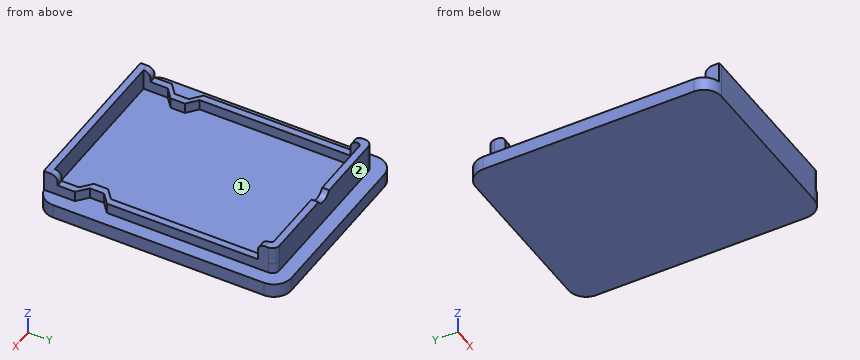
from build123d import *

# Parameters (mm, degrees)
PAD_DEPTH    = 2
PAD001_DEPTH = 1.5
PAD002_DEPTH = 1.5
PAD003_DEPTH = 2.5
SKETCH004_R  = 1.5
POCKET_DEPTH = 5
FILLET_R     = 1
FILLET001_R  = 1
FILLET002_R  = 1


with BuildPart() as part:
    # Sketch → Pad (new body)
    with BuildSketch(Plane.XY):
        with BuildLine():
            Line((-11.5, 17.5), (11.5, 17.5))
            ThreePointArc((14, 15), (13.267767, 16.767767), (11.5, 17.5))
            Line((14, 15), (14, -15))
            ThreePointArc((11.5, -17.5), (13.267767, -16.767767), (14, -15))
            Line((11.5, -17.5), (-11.5, -17.5))
            ThreePointArc((-14, -15), (-13.267767, -16.767767), (-11.5, -17.5))
            Line((-14, -15), (-14, 15))
            ThreePointArc((-11.5, 17.5), (-13.267767, 16.767767), (-14, 15))
        make_face()
    extrude(amount=PAD_DEPTH)

    # Sketch001 (on Face10 of Pad) → Pad001 (join)
    with BuildSketch(Plane.XY.offset(2)):
        with BuildLine():
            Line((-11, 15.5), (11, 15.5))
            ThreePointArc((12, 14.5), (11.707107, 15.207107), (11, 15.5))
            Line((12, 14.5), (12, -8.5))
            Line((12, -8.5), (10.5, -9.76))
            Line((10.5, -9.76), (10.5, -11.79))
            Line((10.5, -11.79), (12, -13.05))
            Line((12, -13.05), (12, -17.44949))
            ThreePointArc((11.5, -17.5), (11.751272, -17.48734), (12, -17.44949))
            Line((-11.5, -17.5), (11.5, -17.5))
            ThreePointArc((-12, -17.44949), (-11.751272, -17.48734), (-11.5, -17.5))
            Line((-12, -13.05), (-12, -17.44949))
            Line((-10.5, -11.79), (-12, -13.05))
            Line((-10.5, -9.76), (-10.5, -11.79))
            Line((-12, -8.5), (-10.5, -9.76))
            Line((-12, 14.5), (-12, -8.5))
            ThreePointArc((-11, 15.5), (-11.707107, 15.207107), (-12, 14.5))
        make_face()
        with BuildLine():
            Line((-11, -16.5), (-11, -13.05))
            Line((-11, -13.05), (-9.5, -11.79))
            Line((-9.5, -11.79), (-9.5, -9.76))
            Line((-9.5, -9.76), (-11, -8.5))
            Line((-11, -8.5), (-11, 14))
            ThreePointArc((-10.5, 14.5), (-10.853553, 14.353553), (-11, 14))
            Line((-10.5, 14.5), (10.5, 14.5))
            ThreePointArc((11, 14), (10.853553, 14.353553), (10.5, 14.5))
            Line((11, 14), (11, -8.5))
            Line((11, -8.5), (9.5, -9.76))
            Line((9.5, -9.76), (9.5, -11.79))
            Line((9.5, -11.79), (11, -13.05))
            Line((11, -13.05), (11, -16.5))
            Line((11, -16.5), (-11, -16.5))
        make_face(mode=Mode.SUBTRACT)
    extrude(amount=PAD001_DEPTH)

    # Sketch002 (on Face26 of Pad001) → Pad002 (join)
    with BuildSketch(Plane.XY.offset(3.5)):
        with BuildLine():
            ThreePointArc((11.5, -17.5), (11.751272, -17.48734), (12, -17.44949))
            Line((12, -16.5), (12, -17.44949))
            Line((12, -15.5), (12, -16.5))
            Line((11, -15.5), (12, -15.5))
            Line((11, -16.5), (11, -15.5))
            Line((11, -16.5), (-11, -16.5))
            Line((-11, -15.5), (-11, -16.5))
            Line((-12, -15.5), (-11, -15.5))
            Line((-12, -16.5), (-12, -15.5))
            Line((-12, -16.5), (-12, -17.44949))
            ThreePointArc((-12, -17.44949), (-11.751272, -17.48734), (-11.5, -17.5))
            Line((-11.5, -17.5), (11.5, -17.5))
        make_face()
    extrude(amount=PAD002_DEPTH)

    # Sketch003 (on Face28 of Pad002) → Pad003 (join)
    with BuildSketch(Plane.XY.offset(3.5)):
        with BuildLine():
            Line((-10.999986, 15.5), (11.000009, 15.5))
            ThreePointArc((12, 14.5), (11.70711, 15.207104), (11.000009, 15.5))
            Line((12, 14.5), (12, 13))
            Line((11, 13), (12, 13))
            Line((11, 14), (11, 13))
            ThreePointArc((11, 14), (10.853553, 14.353553), (10.5, 14.5))
            Line((-10.5, 14.5), (10.5, 14.5))
            ThreePointArc((-10.5, 14.5), (-10.853553, 14.353553), (-11, 14))
            Line((-11, 14), (-11, 13))
            Line((-12, 13), (-11, 13))
            Line((-12, 14.5), (-12, 13))
            ThreePointArc((-10.999986, 15.5), (-11.707102, 15.207112), (-12, 14.5))
        make_face()
    extrude(amount=PAD003_DEPTH)

    # Sketch004 (on Face33 of Pad003) → Pocket (cut)
    with BuildSketch(Plane(origin=(0, 15.5, 0), x_dir=(-1, 0, 0), z_dir=(0, 1, 0))):
        with Locations((0, 6.7)):
            Circle(SKETCH004_R)
    extrude(amount=-POCKET_DEPTH, mode=Mode.SUBTRACT)

    # Fillet
    fillet_edges = [part.edges().sort_by_distance(p)[0] for p in [
        (11.5, -15.5, 5),
    ]]
    fillet(fillet_edges, radius=FILLET_R)

    # Fillet001
    fillet001_edges = [part.edges().sort_by_distance(p)[0] for p in [
        (-11.5, -15.5, 5),
    ]]
    fillet(fillet001_edges, radius=FILLET001_R)

    # Fillet002
    fillet002_edges = [part.edges().sort_by_distance(p)[0] for p in [
        (-11.5, 13, 6),
        (11.5, 13, 6),
    ]]
    fillet(fillet002_edges, radius=FILLET002_R)


solid = part.part
The model under review builds one solid part; all positions refer to its coordinate system, in mm. Face numbers are marked on the shaded views. Coordinates: 2 decimals unless noted, no trailing zeros. Write each loop counter-clockwise with the first axis right and the second up, starting at its lowest first coordinate (ties: lowest second). Pieces come first, ordered by that corner, then holes. Notation, with made-up numbers: (-16.5, -20.75) - (23.5, -20.75) arc R32 cw to (23.5, 14.25) - close; hole circle Ø11 at (-5, 65). An arc over 180 degrees is marked (long way). Answer as a JSON object with one key per item and string values. Group by question number.
1. Add section B-B (x = 3). Give the boundary of the cut face in (y, z), plus the area to 3 significant figures.
2. Add section C-C (y = 7.5). Give the boundary of the cut face in (x, z), plus the area to 3 significant figures.
3. Mouldability with a two-part tool opening along X and no side actions: class the marked faces 1 and 2 as pulls with the +X half, pulls with the -X half, needs draft (parallel to the pull), parting line crosses it, or undercut.
4. Clearance check with flat-ended pins moving along their axes: pin 1 Ø1.5 at (y, z) = (-14.5, 3.5) entering from +X; pin 2 Ø1.5 at (x, z) = (-3.5, 3) entering from +Y; pin 3 Ø2 at (x, y) = (-5.5, 6.5) entering from +Z; pin 4 Ø1.2 at (y, z) = (1.5, 4.5) entering from +X. State where each tip first meets the part, or that it passes through.
5. To check wall thickness, follow probe 1 along X at (y, z) = (10.5, 2.5); probe 2 along Y at (x, z) = (-9.25, 3); probe 3 along Z at (x, y) = (4.75, 13.5). State the ranges of each line that lie inside material, in increasing order.
Findings:
{
 "1": {"outline": "(-17.5, 0) - (17.5, 0) - (17.5, 2) - (15.5, 2) - (15.5, 6) - (14.5, 6) - (14.5, 2) - (-16.5, 2) - (-16.5, 5) - (-17.5, 5) - close", "area": "77.0 mm²"},
 "2": {"outline": "(-14, 0) - (14, 0) - (14, 2) - (12, 2) - (12, 3.5) - (11, 3.5) - (11, 2) - (-11, 2) - (-11, 3.5) - (-12, 3.5) - (-12, 2) - (-14, 2) - close", "area": "59.0 mm²"},
 "3": {"face 1": "undercut", "face 2": "needs draft"},
 "4": {"pin 1": "x = 12", "pin 2": "y = 15.5", "pin 3": "z = 2", "pin 4": "through"},
 "5": {"probe 1": "-12 to -11, 11 to 12", "probe 2": "-17.5 to -16.5, 14.5 to 15.5", "probe 3": "0 to 2"}
}
